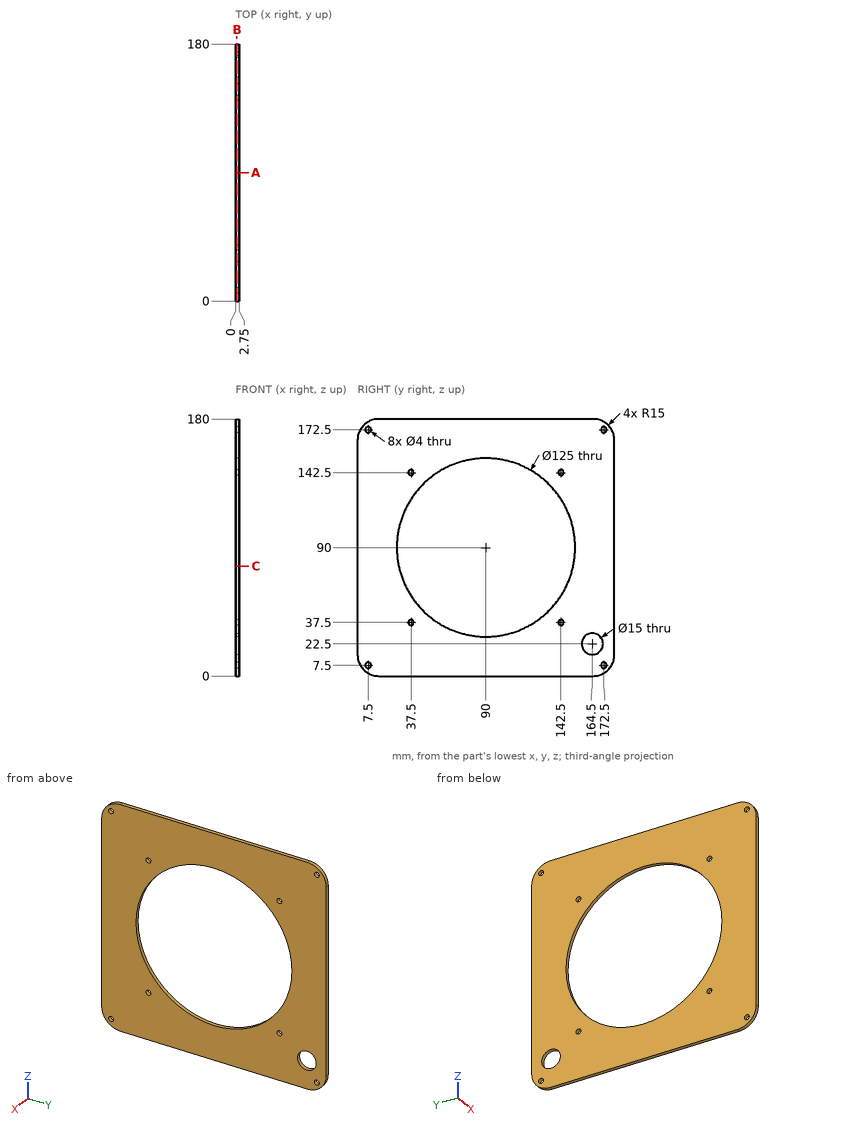
Answer from the drawing. Dimensions are ordinates in mm from the lowest x, y and z of the part. Coordinates: 2 decimals unless noted, no trailing zeros. Write each loop counter-clockwise with the first axis right and the second up, starting at its lowest first coordinate (ties: lowest second). Pieces come first, ordered by that corner, then holes. Notation, with made-up numbers: M -20.75,-26.5 L 7.25,-26.5 A19 cw 7.25,-12.5 Z; hole C 47.25,54 d3. An arc over 180 degrees is marked long. Put each result on its own line as item: value. Start each with the question number.
1. A cutting plane is placed at B-B on x = 0.85. Count the separate pieces of the cut face and the enclosed holes in it, then the cut area to 3 significant figures.
2. A cutting plane is placed at C-C on z = 77. Write down the section's boundary in (x, y), then the cut area to 3 significant figures.
3. Consider line 1 (Y direction, x = 0.3, z = 89.5); line 2 (Z direction, x = 0.8, y = 37.5). Determine where each line is inside the solid, lowest interval first. Write a range as from..to.
4. A cutting plane is placed at A-A on y = 90. Write down the section's boundary in (x, z), then the cut area to 3 significant figures.
Resolved:
1. separate pieces: 1
1. enclosed holes: 10
1. area: 19,700 mm2
2. outline: M 0,0 L 2.75,0 L 2.75,28.87 L 0,28.87 Z; M 0,151.13 L 2.75,151.13 L 2.75,180 L 0,180 Z
2. area: 159 mm2
3. line 1: y = 0..27.5, 152.5..180
3. line 2: z = 0..35.5, 39.5..56.09, 123.91..140.5, 144.5..180
4. outline: M 0,0 L 2.75,0 L 2.75,27.5 L 0,27.5 Z; M 0,152.5 L 2.75,152.5 L 2.75,180 L 0,180 Z
4. area: 151 mm2
